Geometry check sheet. Reference: drawing and pictorial views, mm from the part's lowest x, y, z. Round coordinates to 2 decimals unless told otherwise and drop trailing zeros. Order: outer loops, then holes, each group sorted by start corner. A loop starts at its lowest first (then second) coordinate and runs counter-clockwise, first axis right, second up.
(1) Sectioned sample at A-A, the plane x = 35. Enter the section's corners in (y, z), and give its area (3 significant figures).
(2) Thickness scan on probe 1 along Y at (x, z) = (35, 1); probe 2 along Z at (x, y) = (14.5, 8.25); probe 3 along X at (y, z) = (4.75, 0.85). Record the ranges inside material, lowest first.
(3) Sectioned sample at B-B, the plane y = 5. Enter the section's corners in (x, z), and give its area (3 significant figures).
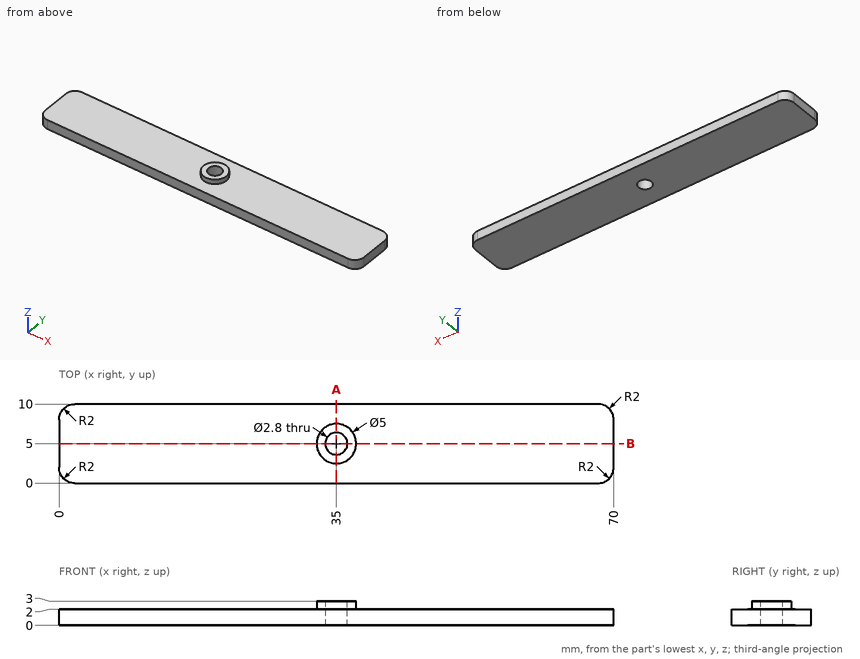
Derived:
1. outline: (0, 0) - (3.6, 0) - (3.6, 3) - (2.5, 3) - (2.5, 2) - (0, 2) - close; (6.4, 0) - (10, 0) - (10, 2) - (7.5, 2) - (7.5, 3) - (6.4, 3) - close
1. area: 16.6 mm2
2. probe 1: y = 0 to 3.6, 6.4 to 10
2. probe 2: z = 0 to 2
2. probe 3: x = 0 to 33.62, 36.38 to 70
3. outline: (0, 0) - (33.6, 0) - (33.6, 3) - (32.5, 3) - (32.5, 2) - (0, 2) - close; (36.4, 0) - (70, 0) - (70, 2) - (37.5, 2) - (37.5, 3) - (36.4, 3) - close
3. area: 137 mm2
